The figure shows three views and two pictorial views of one solid part (mm, origin at its lowest corner). Answer the questions. A direction names the side the tool comes from. Round coordinates to 2 decimals unless told otherwise and drop trailing zeros. Order: outer loops, then holes, each group sorted by start corner. A loop starts at its lowest first (then second) coordinate and runs counter-clockwise, first axis right, second up. Notation, with made-up numbers: (70.25, 15.25) - (115.25, 15.25) arc R21 cw to (115.25, 49.25) - close; hole circle Ø3 at (-9.5, 79). An arc over 180 degrees is marked (long way). Write item = value, one per line.
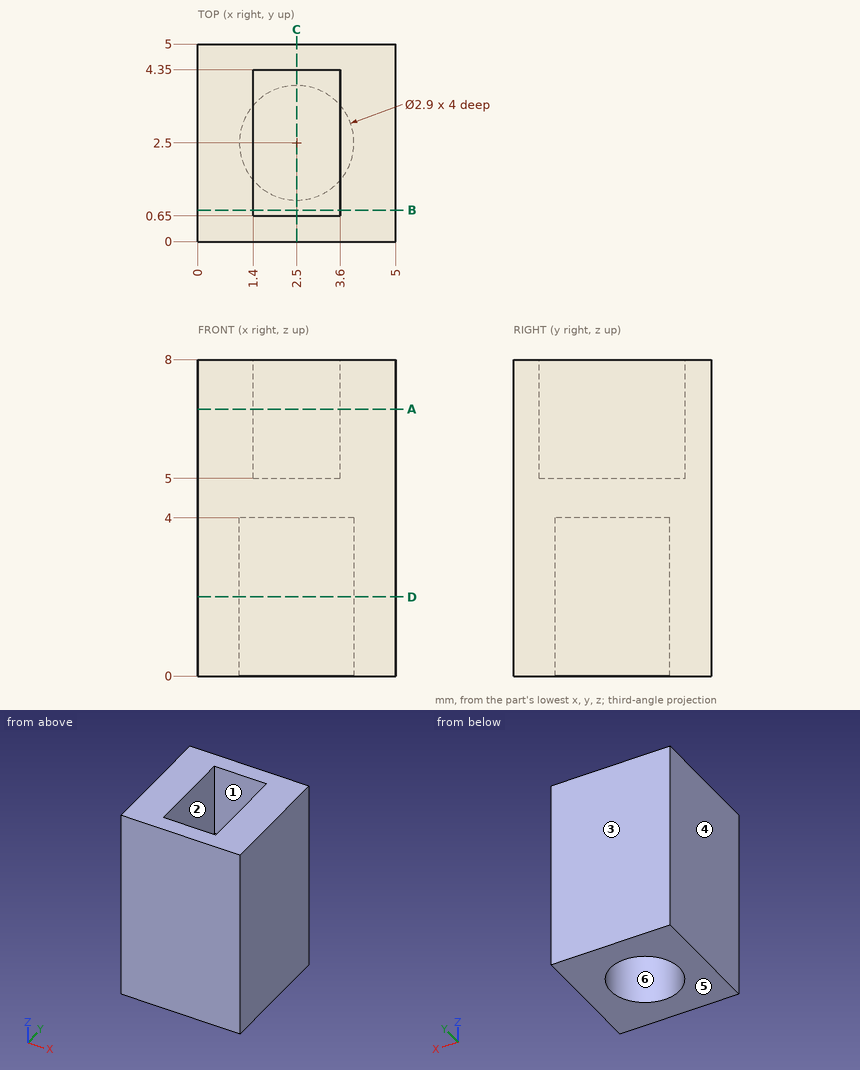
Q1. Determine the mould class of the marked faces 1, 2, 3 and 4 for opening direction X: released by +X, released by -X, zero draft, split by the parting line, or undercut.
Model answer:
face_1 = undercut
face_2 = undercut
face_3 = zero draft
face_4 = released by -X
Q2. Flat-ended cylindrical pins translate along their axes: P1, Ø1.1, axis at x = 2.5, y = 3, coming from the +Z side; P2, Ø2.5, axis at x = 2.5, y = 2.5, coming from the -Z side. Find the tip coordinate at first contact, or state that the pin passes through.
Model answer:
P1 = 5
P2 = 4
Q3. Section D-D on z = 2 is taken. Determine the outline of the cut face in (x, y), then the cut area to 3 significant figures.
Model answer:
outline = (0, 0) - (5, 0) - (5, 5) - (0, 5) - close; hole circle Ø2.9 at (2.5, 2.5)
area = 18.4 mm^2
Q4. Section C-C on x = 2.5 is taken. Determine the outline of the cut face in (y, z).
Model answer:
outline = (0, 0) - (1.05, 0) - (1.05, 4) - (3.95, 4) - (3.95, 0) - (5, 0) - (5, 8) - (4.35, 8) - (4.35, 5) - (0.65, 5) - (0.65, 8) - (0, 8) - close
Q5. Find the intervals of material crossed by line 1 (Y direction, x = 2.5, z = 3.1); line 2 (X direction, y = 3.8, z = 5.5); line 3 (Z direction, x = 2.15, y = 4.05), in increasing order. Write a range as from..to.
Model answer:
line_1 = 0..1.05, 3.95..5
line_2 = 0..1.4, 3.6..5
line_3 = 0..5
Q6. For the marked faces 5 and 6, determine the directions among +Z, -Z, +X, -X, +Y, -Y from which every point of the face is accessible in a straight line to the end or side of a thin tool.
Model answer:
face_5 = -Z, +X, -X, +Y, -Y
face_6 = -Z
Q7. Section A-A on z = 6.75 is taken. Determine the outline of the cut face in (x, y), then the cut area to 3 significant figures.
Model answer:
outline = (0, 0) - (5, 0) - (5, 5) - (0, 5) - close; hole (1.4, 0.65) - (3.6, 0.65) - (3.6, 4.35) - (1.4, 4.35) - close
area = 16.9 mm^2
Q8. Section B-B on y = 0.8 is taken. Determine the outline of the cut face in (x, z), then the cut area to 3 significant figures.
Model answer:
outline = (0, 0) - (5, 0) - (5, 8) - (3.6, 8) - (3.6, 5) - (1.4, 5) - (1.4, 8) - (0, 8) - close
area = 33.4 mm^2
